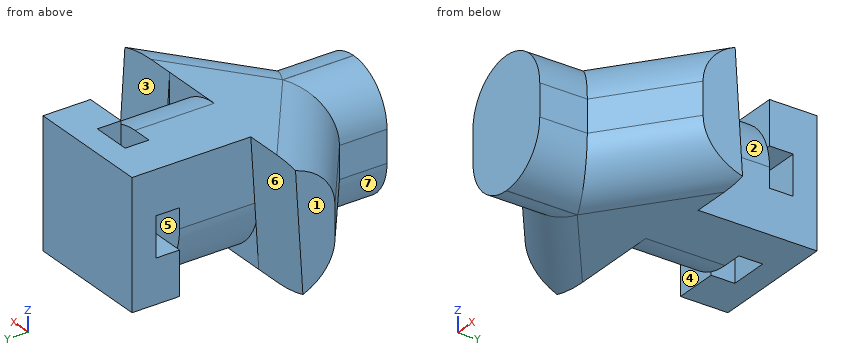
from build123d import *

# Parameters (mm, degrees)
PAD_DEPTH       = 8
PAD001_DEPTH    = 5
PAD002_DEPTH    = 4
PAD003_DEPTH    = 4
SKETCH004_W     = 8
SKETCH004_H     = 8
PAD004_DEPTH    = 3
SKETCH005_W     = 2.5
SKETCH005_H     = 1.5
POCKET_DEPTH    = 8.001
SKETCH006_W     = 1.5
SKETCH006_H     = 2.5
POCKET001_DEPTH = 12.001
FILLET_R        = 2.99
FILLET001_R     = 2.99


with BuildPart() as part:
    # Sketch → Pad (new body)
    with BuildSketch(Plane.XY):
        Polygon((-8, 0), (8, 0), (8, -2), (3, -5.8), (3, -8.8), (-3, -8.8), (-3, -5.8), (-8, -2), align=None)
    extrude(amount=PAD_DEPTH)

    # Sketch001 (on Face2 of Pad) → Pad001 (join)
    with BuildSketch(Plane(origin=(0, 0, 0), x_dir=(-1, 0, 0), z_dir=(0, 1, 0))):
        with BuildLine():
            Line((-4, 4), (-4, 0))
            Line((-4, 0), (0, 0))
            ThreePointArc((0, 0), (2.828427, 1.171573), (4, 4))
            Line((4, 4), (4, 8))
            Line((4, 8), (0, 8))
            ThreePointArc((0, 8), (-2.828427, 6.828427), (-4, 4))
        make_face()
    extrude(amount=PAD001_DEPTH)

    # Sketch002 (on Face13 of Pad001) → Pad002 (join)
    with BuildSketch(Plane.YZ.offset(4)):
        Polygon((0, 0), (0, 8), (0.5, 0), align=None)
    extrude(amount=PAD002_DEPTH)

    # Sketch003 (on Face6 of Pad002) → Pad003 (join)
    with BuildSketch(Plane(origin=(-4, 0, 0), x_dir=(0, -1, 0), z_dir=(-1, 0, 0))):
        Polygon((0, 0), (0, 8), (-0.5, 8), align=None)
    extrude(amount=PAD003_DEPTH)

    # Sketch004 (on Face7 of Pad003) → Pad004 (join)
    with BuildSketch(Plane(origin=(0, 5, 0), x_dir=(-1, 0, 0), z_dir=(0, 1, 0))):
        with Locations((0, 4)):
            Rectangle(SKETCH004_W, SKETCH004_H)
    extrude(amount=PAD004_DEPTH)

    # Sketch005 (on Face20 of Pad004) → Pocket (cut, through all)
    with BuildSketch(Plane.XY.offset(8)):
        with Locations((0, 5.75)):
            Rectangle(SKETCH005_W, SKETCH005_H)
    extrude(amount=-POCKET_DEPTH, mode=Mode.SUBTRACT)

    # Sketch006 (on Face9 of Pocket) → Pocket001 (cut, through all)
    with BuildSketch(Plane.YZ.offset(4)):
        with Locations((5.75, 4)):
            Rectangle(SKETCH006_W, SKETCH006_H)
    extrude(amount=-POCKET001_DEPTH, mode=Mode.SUBTRACT)

    # Fillet
    fillet_edges = [part.edges().sort_by_distance(p)[0] for p in [
        (-3, -7.3, 8),
        (3, -7.3, 8),
        (-3, -7.3, 0),
        (3, -7.3, 0),
    ]]
    fillet(fillet_edges, radius=FILLET_R)

    # Fillet001
    fillet001_edges = [part.edges().sort_by_distance(p)[0] for p in [
        (-5.5, -3.9, 8),
        (5.5, -3.9, 8),
        (-5.5, -3.9, 0),
        (5.5, -3.9, 0),
    ]]
    fillet(fillet001_edges, radius=FILLET001_R)


solid = part.part
Read the model definition and answer for the solid it produces. Units are mm, in the model's axes. Face numbers are marked on the shaded views. A direction names the side the tool comes from. Give positions to 0.01 mm unless a question says otherwise; leave off trailing zeros. Write each loop counter-clockwise with the first axis right and the second up, starting at its lowest first coordinate (ties: lowest second). Pieces come first, ordered by that corner, then holes. Notation, with made-up numbers: (49, 28.25) - (106, 28.25) arc R21 ccw to (106, 52.25) - close; hole circle Ø4 at (21.25, 62). An arc over 180 degrees is marked (long way). Answer in a Markdown table with one row per item. Add a question column.
Item 1: Section C-C, the plane z = 1.75 is taken. Write down the section's boundary in (x, y).
Item 2: Flat-ended cylindrical pins translate along their axes: P1, Ø6, axis at x = 6, y = -6, coming from the +Z side; P2, Ø2, axis at x = 5, y = -3, coming from the +Z side; P3, Ø1, axis at x = -5, z = 7, coming from the +Y side. Find the tip coordinate at first contact, or state that the pin passes through.
Item 3: Find the intervals of material crossed by L1, parallel to Y at x = -0.5, z = 4; L2, parallel to X at y = 6, z = 7.25; L3, parallel to Z at x = -2.25, y = 6.25, in increasing order.
Item 4: A tool of negligible diameter and unlimited length cuts with its end or side. For the marked faces 4, 5, 6 and 7, from which of +Z, -Z, +X, -X, +Y, -Y can it reach the whole face along a straight path? Write none if from no direction.
Item 5: Determine the mould class of the marked faces 1, 2 and 3 for opening direction Y: pulls with the +Y half, pulls with the -Y half, needs draft (parallel to the pull), parting line crosses it, or undercut.
Item 6: Section D-D, the plane y = 1.5 is taken. Write down the section's boundary in (x, z).
Recorded:
| question | item | result |
|---|---|---|
| 1 | outline | (-8, -1.66) - (-2.73, -5.67) - (-2.73, -8.8) - (2.73, -8.8) - (2.73, -5.67) - (8, -1.66) - (8, 0.39) - (4, 0.39) - (4, 8) - (-4, 8) - (-4, 5) - (-3.31, 5) - (-3.31, 0) - (-4, 0) - (-4, 0.11) - (-8, 0.11) - close; hole (-1.25, 5) - (1.25, 5) - (1.25, 6.5) - (-1.25, 6.5) - close |
| 2 | P1 | stops at z = 7.26 |
| 2 | P2 | stops at z = 7.84 |
| 2 | P3 | stops at y = 0.47 |
| 3 | L1 | y = -8.8 to 5, 6.5 to 8 |
| 3 | L2 | x = -4 to -1.25, 1.25 to 4 |
| 3 | L3 | z = 0 to 2.75, 5.25 to 8 |
| 4 | face 4 | -Z, -X |
| 4 | face 5 | none |
| 4 | face 6 | -Z, -X, +Y |
| 4 | face 7 | -Z, -X, -Y |
| 5 | face 1 | needs draft |
| 5 | face 2 | undercut |
| 5 | face 3 | pulls with the +Y half |
| 6 | outline | (-4, 4) arc R4 ccw to (0, 0) - (4, 0) - (4, 4) arc R4 ccw to (0, 8) - (-4, 8) - close |
